```python
from build123d import *

# Parameters (mm, degrees)
F0_W     = 48
F0_H     = 34
F1_DEPTH = 5
F2_R     = 1.5
F3_DEPTH = 5
F4_W     = 24
F4_H     = 24
F5_DEPTH = 30
F6_W     = 20
F6_H     = 20
F7_DEPTH = 20


with BuildPart() as f1:
    # F0 (on Top) → F1 (new body)
    with BuildSketch(Plane.XY):
        Rectangle(F0_W, F0_H)
    extrude(amount=-F1_DEPTH)

    # F2 (on face) → F3 (cut)
    with BuildSketch(Plane.XY):
        with Locations((-19.5, 0)):
            Circle(F2_R)
        with BuildLine():
            ThreePointArc((21, 0), (19.5, 1.5), (18, 0))
            ThreePointArc((18, 0), (19.5, -1.5), (21, 0))
        make_face()
    extrude(amount=-F3_DEPTH, mode=Mode.SUBTRACT)

    # F4 (on face) → F5 (join)
    with BuildSketch(Plane.XY):
        Rectangle(F4_W, F4_H)
    extrude(amount=F5_DEPTH)

    # F6 (on face) → F7 (cut)
    with BuildSketch(Plane.XY.offset(30)):
        Rectangle(F6_W, F6_H)
    extrude(amount=-F7_DEPTH, mode=Mode.SUBTRACT)


solid = f1.part
```
Source: CAD feature listing. Evaluate the final solid. Frame: model axes, mm. A direction names the side the tool comes from. Give positions to 0.01 mm unless a question says otherwise; leave off trailing zeros. Loops run counter-clockwise (first coordinate to the right, second up) from the corner with the lowest first, then second, coordinate; pieces in that order, holes last. Notation, with made-up numbers: M 67.5,6.5 L 105.5,6.5 A30 cw 105.5,32.5 Z; hole C 12.5,52 d1. An arc over 180 degrees is marked long. Put each result on its own line as item: value.
Q1. Reachability of faces 1 (the flat face through (12, 0, 15)), 2 (the flat face through (-12, 0, 15)), 3 (the flat face through (-10, 0, 20)) from +Z, -Z, +X, -X, +Y, -Y: full face, straight path, thin tool, end or side. Return the list, or none.
Response values:
face 1: +Z, +X, +Y, -Y
face 2: +Z, -X, +Y, -Y
face 3: +Z
Q2. Mould query, pull axis Y, two halves, no side actions, for faces 4 (the flat face through (0, -12, 15)), 5 (the flat face through (0, 0, -5)), 6 (the flat face through (0, 10, 20)). Classes: released by +Y, released by -Y, zero draft, split by the parting line, or undercut.
Response values:
face 4: released by -Y
face 5: zero draft
face 6: undercut
Q3. Section D-D (y = 3.5). Return the cut outline in (x, z).
Response values:
outline: M -24,-5 L 24,-5 L 24,0 L 12,0 L 12,30 L 10,30 L 10,10 L -10,10 L -10,30 L -12,30 L -12,0 L -24,0 Z
Q4. Section A-A (z = 19). Return the cut outline in (x, y), and give its area (3 significant figures).
Response values:
outline: M -12,-12 L 12,-12 L 12,12 L -12,12 Z; hole M -10,-10 L 10,-10 L 10,10 L -10,10 Z
area: 176 mm²
Q5. Line query: probe 1 along X at (y, z) = (7.5, 26); probe 2 along Y at (x, z) = (-19.5, -3.9). Output: solid intervals per line, ascending. Write a range as [from, to].
Response values:
probe 1: x = [-12, -10], [10, 12]
probe 2: y = [-17, -1.5], [1.5, 17]
Q6. Section C-C (x = -19.5). Return the cut outline in (y, z).
Response values:
outline: M -17,-5 L -1.5,-5 L -1.5,0 L -17,0 Z; M 1.5,-5 L 17,-5 L 17,0 L 1.5,0 Z
Q7. Pin query (flat end, axial travel): P1, Ø6, axis at y = 7.5, z = 18.5, coming from the +X side; P2, Ø2.5, axis at x = 19.5, y = 0, coming from the -Z side; P3, Ø16, axis at y = -3, z = 16, coming from the -X side; P4, Ø16, axis at x = -4.5, y = -2.5, coming from the +Z side. Return the tip coordinate at first contact, or that it passes through.
Response values:
P1: stops at x = 12
P2: passes through
P3: stops at x = -12
P4: stops at z = 30
Q8. Section B-B (y = 0). Return the cut outline in (x, z), and give its area (3 significant figures).
Response values:
outline: M -24,-5 L -21,-5 L -21,0 L -24,0 Z; M -18,-5 L 18,-5 L 18,0 L 12,0 L 12,30 L 10,30 L 10,10 L -10,10 L -10,30 L -12,30 L -12,0 L -18,0 Z; M 21,-5 L 24,-5 L 24,0 L 21,0 Z
area: 530 mm²
